Autodesk Inventor part; units mm, degrees
ref_plane "YZ Plane" through (0, 0, 0) normal (1, 0, 0) x (0, 1, 0)
ref_plane "XZ Plane" through (0, 0, 0) normal (0, 1, 0) x (-1, 0, 0)
ref_plane "XY Plane" through (0, 0, 0) normal (0, 0, 1) x (1, 0, 0)
sketch "Sketch2" plane through (0, 0, 0) normal (0, 1, 0) x (-1, 0, 0)
  line L0 (-54, -130.3675) -> (-130.3675, -54)
  line L1 (-130.3675, -54) -> (-130.3675, 54)
  line L2 (-130.3675, 54) -> (-54, 130.3675)
  line L3 (-54, 130.3675) -> (54, 130.3675)
  line L4 (54, 130.3675) -> (130.3675, 54)
  line L5 (130.3675, 54) -> (130.3675, -54)
  line L6 (130.3675, -54) -> (54, -130.3675)
  line L7 (54, -130.3675) -> (-54, -130.3675)
  line L8 (57646.2618, 0) -> (-57646.2618, 0)
  line L9 (-39, -121.3675) -> (39, -121.3675)
  line L10 (39, -121.3675) -> (39, -90.3675)
  line L11 (39, -90.3675) -> (-39, -90.3675)
  line L12 (-39, -90.3675) -> (-39, -121.3675)
  line L13 (90.3675, -39) -> (121.3675, -39)
  line L14 (90.3675, 39) -> (90.3675, -39)
  line L15 (121.3675, -39) -> (121.3675, 39)
  line L16 (121.3675, 39) -> (90.3675, 39)
  line L17 (39, 90.3675) -> (39, 121.3675)
  line L18 (-39, 90.3675) -> (39, 90.3675)
  line L19 (39, 121.3675) -> (-39, 121.3675)
  line L20 (-39, 121.3675) -> (-39, 90.3675)
  line L21 (-90.3675, 39) -> (-121.3675, 39)
  line L22 (-90.3675, -39) -> (-90.3675, 39)
  line L23 (-121.3675, 39) -> (-121.3675, -39)
  line L24 (-121.3675, -39) -> (-90.3675, -39)
  circle A0 centre (-13.775, -86.8675) radius 1.6
  line L25 (0, -3770.9416) -> (0, 3770.9416)
  circle A1 centre (-13.775, -64.5175) radius 1.6
  circle A2 centre (13.775, -86.8675) radius 1.6
  circle A3 centre (13.775, -64.5175) radius 1.6
  circle A4 centre (86.8675, -13.775) radius 1.6
  circle A5 centre (86.8675, 13.775) radius 1.6
  circle A6 centre (64.5175, -13.775) radius 1.6
  circle A7 centre (64.5175, 13.775) radius 1.6
  circle A8 centre (13.775, 86.8675) radius 1.6
  circle A9 centre (-13.775, 86.8675) radius 1.6
  circle A10 centre (13.775, 64.5175) radius 1.6
  circle A11 centre (-13.775, 64.5175) radius 1.6
  circle A12 centre (-86.8675, 13.775) radius 1.6
  circle A13 centre (-86.8675, -13.775) radius 1.6
  circle A14 centre (-64.5175, 13.775) radius 1.6
  circle A15 centre (-64.5175, -13.775) radius 1.6
  line L26 (-14.2258, -50.4297) -> (-15.64, -49.0154)
  line L27 (-15.64, -49.0154) -> (-9.9831, -43.3586)
  line L28 (-9.9831, -43.3586) -> (-8.5689, -44.7728)
  line L29 (-8.5689, -44.7728) -> (-14.2258, -50.4297)
  line L30 (-57646.2618, 0) -> (57646.2618, 0)
  circle A16 centre (20.9157, -74.2574) radius 1.6
  line L31 (0, 3770.9416) -> (0, -3770.9416)
  line L32 (-48.6843, -48.6843) -> (48.6843, 48.6843)
  line L33 (-48.6843, -48.6843) -> (89.0157, -48.6843) construction
  line L34 (16.6877, -16.6877) -> (-16.6877, 16.6877)
  line L35 (-50.4297, -14.2258) -> (-49.0154, -15.64)
  line L36 (-49.0154, -15.64) -> (-43.3586, -9.9831)
  line L37 (-43.3586, -9.9831) -> (-44.7728, -8.5689)
  line L38 (-44.7728, -8.5689) -> (-50.4297, -14.2258)
  line L39 (50.4297, 14.2258) -> (49.0154, 15.64)
  line L40 (49.0154, 15.64) -> (43.3586, 9.9831)
  line L41 (43.3586, 9.9831) -> (44.7728, 8.5689)
  line L42 (44.7728, 8.5689) -> (50.4297, 14.2258)
  line L43 (9.9831, 43.3586) -> (8.5689, 44.7728)
  line L44 (14.2258, 50.4297) -> (15.64, 49.0154)
  line L45 (15.64, 49.0154) -> (9.9831, 43.3586)
  line L46 (8.5689, 44.7728) -> (14.2258, 50.4297)
  line L47 (-32.0673, -65.4427) -> (-42.6739, -54.8361)
  line L48 (-42.6739, -54.8361) -> (-36.3099, -48.4722)
  line L49 (-36.3099, -48.4722) -> (-25.7033, -59.0788)
  line L50 (-25.7033, -59.0788) -> (-32.0673, -65.4427)
  line L51 (-56.9575, -40.5526) -> (-65.4427, -32.0673)
  line L52 (-65.4427, -32.0673) -> (-60.1394, -26.764)
  line L53 (-60.1394, -26.764) -> (-51.6542, -35.2493)
  line L54 (-51.6542, -35.2493) -> (-56.9575, -40.5526)
  line L55 (20.1657, -61.8405) -> (20.1657, -64.5905) construction
  line L56 (19.4157, -62.5905) -> (19.4157, -63.8405)
  line L57 (20.9157, -63.8405) -> (20.9157, -62.5905)
  arc A17 (20.9157, -62.5905) -> (19.4157, -62.5905) centre (20.1657, -62.5905) ccw
  arc A18 (19.4157, -63.8405) -> (20.9157, -63.8405) centre (20.1657, -63.8405) ccw
  arc A19 (62.5905, 20.9157) -> (62.5905, 19.4157) centre (62.5905, 20.1657) ccw
  line L58 (63.8405, 20.9157) -> (62.5905, 20.9157)
  line L59 (62.5905, 19.4157) -> (63.8405, 19.4157)
  arc A20 (63.8405, 19.4157) -> (63.8405, 20.9157) centre (63.8405, 20.1657) ccw
  line L60 (61.8405, 20.1657) -> (64.5905, 20.1657) construction
  arc A21 (-20.9157, 62.5905) -> (-19.4157, 62.5905) centre (-20.1657, 62.5905) ccw
  line L61 (-20.9157, 63.8405) -> (-20.9157, 62.5905)
  line L62 (-19.4157, 62.5905) -> (-19.4157, 63.8405)
  arc A22 (-19.4157, 63.8405) -> (-20.9157, 63.8405) centre (-20.1657, 63.8405) ccw
  line L63 (-20.1657, 61.8405) -> (-20.1657, 64.5905) construction
  arc A23 (-62.5905, -20.9157) -> (-62.5905, -19.4157) centre (-62.5905, -20.1657) ccw
  line L64 (-63.8405, -20.9157) -> (-62.5905, -20.9157)
  line L65 (-62.5905, -19.4157) -> (-63.8405, -19.4157)
  arc A24 (-63.8405, -19.4157) -> (-63.8405, -20.9157) centre (-63.8405, -20.1657) ccw
  line L66 (-61.8405, -20.1657) -> (-64.5905, -20.1657) construction
  circle A25 centre (0, 128.0141) radius 1.6
  circle A26 centre (-128.0141, 0) radius 1.6
  circle A27 centre (0, -128.0141) radius 1.6
  circle A28 centre (128.0141, 0) radius 1.6
  circle A29 centre (5.8021, -56.3462) radius 1.6
  circle A30 centre (74.2574, 20.9157) radius 1.6
  circle A31 centre (56.3462, 5.8021) radius 1.6
  circle A32 centre (-20.9157, 74.2574) radius 1.6
  circle A33 centre (-5.8021, 56.3462) radius 1.6
  circle A34 centre (-74.2574, -20.9157) radius 1.6
  circle A35 centre (-56.3462, -5.8021) radius 1.6
  point P0 (0, 0)
  point P1 (0, 0)
  point P2 (0, 0)
  point P3 (0, 0)
  point P4 (0, 0)
  point P5 (0, 0)
  point P6 (0, 0)
  point P7 (0, 0)
  point P8 (20.1657, -63.2155)
  point P9 (63.2155, 20.1657)
  point P10 (-20.1657, 63.2155)
  point P11 (-63.2155, -20.1657)
  dimension "d5" = 9
  dimension "d6" = 31
  dimension "d7" = 15
  dimension "d8" = 15
  dimension "d11" = 360
  dimension "d13" = 78
  dimension "d14" = 13.775
  dimension "d16" = 3.5
  dimension "d18" = 22.35
  dimension "d21" = 360
  dimension "d24" = 2
  dimension "d25" = 8
  dimension "d29" = 3.2
  dimension "d41" = 3.2
  dimension "d48" = 137.7
  dimension "d49" = 45
  dimension "d50" = 47.2
  dimension "d51" = 23.6
  dimension "d52" = 9
  dimension "d53" = 15
  dimension "d56" = 68.95
  dimension "d57" = 23.6
  dimension "d58" = 68.95
  dimension "d59" = 23.6
  dimension "d60" = 7.5
  dimension "d61" = 12
  dimension "d62" = 2.75
  dimension "d63" = 1.5
  dimension "d66" = 360
  dimension "d70" = 3.2
  dimension "d73" = 360
  dimension "d83" = 3.2
  dimension "d86" = 360
extrude "Extrusion5" add sketch "Sketch2" along normal blind 3 contours L0 L1 L8 A26 L23 L24 L22 L25 L11 L12 L9 A27 L7 | L25 A27 L9 L10 L11 L8 L14 L13 L15 A28 L5 L6 L7 | L1 L2 L3 L25 A25 L19 L20 L18 L8 L22 L21 L23 A26 | A27 L25 | L25 A27 | A26 L8 | L8 A26 | L8 A28 L15 L16 L14 L25 L18 L17 L19 A25 L3 L4 L5 | A28 L8 | L8 A28 | A25 L25 | L25 A25
equation "\"d8\" = d7"
properties part number "Base"
For this review, take the finished solid that the model builds, in its own axes (mm). A direction names the side the tool comes from. Round coordinates to 2 decimals unless told otherwise and drop trailing zeros. Loops run counter-clockwise (first coordinate to the right, second up) from the corner with the lowest first, then second, coordinate; pieces in that order, holes last. Notation, with made-up numbers: (-9.5, -30.75) - (26.5, -30.75) arc R6 ccw to (26.5, -22.75) - close; hole circle Ø3 at (59, 25.5). An arc over 180 degrees is marked (long way). Put each result on its own line as item: value. Start each with the question number.
1. Consider section C-C on y = 0.5. State how many separate pieces and enclosed holes the cut face has, plus the area to 3 significant figures.
2. For faces 1 (the flat face through (-47.562, 1.479, 11.358)), 2 (the flat face through (-91.65, 1.48, 92.72)), list the 3-axis set-ups (+Z, -Z, +X, -X, +Y, -Y) from which the entire face can be reached by the end or side of a thin tool; tool diameter is ignored.
3. Consider section D-D on z = -80.5. State the section outline as (x, y) points.
4. Consider section A-A on x = -112. State the section outline as (y, z) points.
5. Consider section B-B on x = 108. State the section outline as (y, z) points, plus the area to 3 significant figures.
6. Insertion check: P1, Ø2.5, axis at x = 20.92, z = 74.26, coming from the +Y side; P2, Ø1.4, axis at x = 63.5, y = 1, coming from the -Z side; P3, Ø1.5, axis at y = 2, z = -102, coming from the -X side; P4, Ø1.5, axis at x = 99.5, y = 2, coming from the +Z side. Each pin has a flat end and moves straight along its axis. Give the tip position at first contact, or say it passes through.
7. For probe 1 along X at (y, z) = (1.9, 0); probe 2 along Z at (x, y) = (32, 2.45), list the stretches that pass through material, from the lowest coordinate up. Write a range as [from, to].
8. Mouldability with a two-part tool opening along Z and no side actions: class faces 3 (the flat face through (2, 0, 2)), 4 (the flat face through (92.72, 1.48, 91.65)), 5 (the flat face through (12.851, 1.479, -46.227)) as +Z half, -Z half, draft (parallel to the pull), parting line (faces both ways), or undercut.
Result sheet:
1. separate pieces: 1
1. enclosed holes: 38
1. area: 46,200 mm^2
2. face 1: +Y, -Y
2. face 2: +Z, -X, +Y, -Y
3. outline: (-103.87, 0) - (103.87, 0) - (103.87, 3) - (-103.87, 3) - close
4. outline: (0, -72.37) - (3, -72.37) - (3, -39) - (0, -39) - close; (0, 39) - (3, 39) - (3, 72.37) - (0, 72.37) - close
5. outline: (0, -76.37) - (3, -76.37) - (3, -39) - (0, -39) - close; (0, 39) - (3, 39) - (3, 76.37) - (0, 76.37) - close
5. area: 224 mm^2
6. P1: through
6. P2: z = -121.57
6. P3: x = -83.12
6. P4: z = 85.62
7. probe 1: [-130.37, -121.37], [-90.37, 90.37], [121.37, 130.37]
7. probe 2: [-130.37, -121.37], [-90.37, -65.38], [-52.78, 90.37], [121.37, 130.37]
8. face 3: draft
8. face 4: +Z half
8. face 5: undercut
